Work out the finished part from the listing and answer in its coordinate system (mm). A direction names the side the tool comes from. Round coordinates to 2 decimals unless told otherwise and drop trailing zeros. Loops run counter-clockwise (first coordinate to the right, second up) from the corner with the lowest first, then second, coordinate; pieces in that order, holes last. Notation, with made-up numbers: (61, 26.25) - (66, 26.25) arc R21 cw to (66, 42.25) - close; hole circle Ø5 at (44, 19). An arc over 180 degrees is marked (long way). Use CSV: the item, a comma, the result in double quotes. Start each with the question number.
from build123d import *

# Parameters (mm, degrees)
BOSS_EXTRUDE1_DEPTH     = 22
BOSS_EXTRUDE3_START     = -5
BOSS_EXTRUDE3_OUTLINE_R = 1.5
BOSS_EXTRUDE3_DEPTH     = 5
CHAMFER2_SIZE           = 1
CHAMFER3_SIZE           = 7
CHAMFER3_SIZE2          = 2


# Read off the part's stored shape, not the designer's step: Boss-Extrude3
with BuildPart() as part:
    # Sketch1 → Boss-Extrude1 (new body)
    with BuildSketch(Plane(origin=(0, 0, 0), x_dir=(1, 0, 0), z_dir=(0, 1, 0))):
        with BuildLine():
            Line((0, -16.5), (0, -8.075))
            ThreePointArc((3.5438e-13, -8.075), (-5.709887258081245, -5.709887258081495), (-8.075, 1.03e-15))
            Line((-8.075, 0), (-16.5, 0))
            Line((-16.5, 0), (-24.5, -9.8e-16))
            Line((-24.5, -9.8e-16), (-24.5, -5.000000000000001))
            Line((-24.5, -5.000000000000001), (-15.724185193516389, -5.000000000000001))
            ThreePointArc((-15.724185193516387, -5), (-9.740379869388931, -13.318220601867306), (3.5527e-13, -16.5))
        make_face()
        with BuildLine():
            Line((24.5, -9.8e-16), (16.5, 0))
            Line((16.5, 0), (8.075, 0))
            ThreePointArc((8.075, 3.34e-15), (5.709887258081497, -5.709887258081244), (3.5438e-13, -8.075))
            Line((0, -8.075), (0, -16.5))
            ThreePointArc((3.5527e-13, -16.5), (9.74037986938922, -13.3182206018671), (15.724185193516387, -5.000000000000004))
            Line((15.724185193516389, -5.000000000000001), (24.5, -5.000000000000001))
            Line((24.5, -5.000000000000001), (24.5, -9.8e-16))
        make_face()
    extrude(amount=-BOSS_EXTRUDE1_DEPTH)

    # Boss-Extrude3 outline → Boss-Extrude3 (cut)
    with BuildSketch(Plane.XY.offset(5.000000000000001).offset(BOSS_EXTRUDE3_START)):
        with Locations((20.5, -18)):
            Circle(BOSS_EXTRUDE3_OUTLINE_R)
        with Locations((20.5, -4)):
            Circle(BOSS_EXTRUDE3_OUTLINE_R)
        with Locations((-20.5, -4)):
            Circle(BOSS_EXTRUDE3_OUTLINE_R)
        with Locations((-20.5, -18)):
            Circle(BOSS_EXTRUDE3_OUTLINE_R)
    extrude(amount=BOSS_EXTRUDE3_DEPTH, mode=Mode.SUBTRACT)

    # Chamfer2
    chamfer2_edges = [part.edges().sort_by_distance(p)[0] for p in [
        (-22, -18, 5.000000000000001),
        (19, -4, 5.000000000000001),
        (19, -18, 5.000000000000001),
        (-22, -4, 5.000000000000001),
    ]]
    chamfer(chamfer2_edges, length=CHAMFER2_SIZE)

    # Chamfer3
    chamfer3_edges = [part.edges().sort_by_distance(p)[0] for p in [
        (1.54e-15, -22, 8.075),
    ]]
    chamfer3_side = [part.faces().sort_by_distance(p)[0] for p in [
        (2.05e-15, -11, 8.075),
    ]]
    chamfer(chamfer3_edges, length=CHAMFER3_SIZE, length2=CHAMFER3_SIZE2, reference=chamfer3_side[0])

    # Sketch4 → Cut-Revolve1 (revolve, cut)
    with BuildSketch(Plane(origin=(0, 0, 0), x_dir=(-1, 0, -1.2e-16), z_dir=(1.2e-16, 0, -1))):
        with BuildLine():
            Line((-9.575, 0.4703111185771576), (-9.575, -1.4999999999999998))
            ThreePointArc((-9.575, -1.4999999999999998), (-7.014339828220178, -2.560660171779821), (-8.075, 0))
            Line((-8.075, 0), (-9.575, 0.4703111185771576))
        make_face()
    revolve(axis=Axis((4.3e-16, 1.8602118411515838, 0), (-1.7e-16, -1, 0)), mode=Mode.SUBTRACT)


solid = part.part
Item 1: The mould has two halves that part along X. Classify faces 3 (the flat face through (0, 0, 10)), 4 (the conical face through (0.195, -17.771, 8.865)), 5 (the flat face through (24.5, -11, 3)): pulls with the +X half, pulls with the -X half, needs draft (parallel to the pull), parting line crosses it, or undercut.
Item 2: A cutting plane is placed at B-B (x = 20.5). Determine the outline of the cut face in (y, z), plus the area to 3 significant figures.
Item 3: Find the intervals of material crossed by probe 1 along Y at (x, z) = (-20.5, 3.1); probe 2 along Z at (x, y) = (19, -7); probe 3 along X at (y, z) = (-1, 6), in increasing order. Write a range as [from, to].
Item 4: A cutting plane is placed at D-D (x = -17.5). Determine the outline of the cut face in (y, z), plus the area to 3 significant figures.
Item 5: Which of the six approach directions +Z, -Z, +X, -X, +Y, -Y give full straight-line access (tool end or side, diameter ignored) to faces 1 (the flat face through (20, -11, 5)), 2 (the flat face through (0, -22, 12))?
Item 6: A cutting plane is placed at C-C (y = -9.25). Determine the outline of the cut face in (x, z) (3 decimals).
Item 7: Each of these flat-tipped pins is pushed along its axis until it touches: pin 1 Ø3.5 at (x, y) = (20.5, -18) entering from +Z; pin 2 Ø6 at (x, y) = (-15.5, -7.5) entering from +Z; pin 3 Ø9.5 at (x, y) = (-19, -16) entering from +Z. Where does it stop, or does it pass through?
Item 8: A cutting plane is placed at A-A (y = -4). Determine the outline of the cut face in (x, z) (3 decimals).
Result sheet:
1,face 3,"needs draft"
1,face 4,"undercut"
1,face 5,"pulls with the +X half"
2,outline,"(-22, 0) - (-19.5, 0) - (-19.5, 4) - (-20.5, 5) - (-22, 5) - close; (-16.5, 0) - (-5.5, 0) - (-5.5, 4) - (-6.5, 5) - (-15.5, 5) - (-16.5, 4) - close; (-2.5, 0) - (0, 0) - (0, 5) - (-1.5, 5) - (-2.5, 4) - close"
2,area,"78.0 mm^2"
3,probe 1,"[-22, -19.5], [-16.5, -5.5], [-2.5, 0]"
3,probe 2,"[0, 5]"
3,probe 3,"[-15.37, -7.46], [7.46, 15.37]"
4,outline,"(-22, 0) - (0, 0) - (0, 5) - (-22, 5) - close"
4,area,"110 mm^2"
5,face 1,"+Z, +X, +Y, -Y"
5,face 2,"+Z, -Z, +X, -X, -Y"
6,outline,"(-24.5, 0) - (-8.075, 0) arc R8.075 cw to (8.075, 0) - (24.5, 0) - (24.5, 5) - (15.724, 5) arc R16.5 ccw to (-15.724, 5) - (-24.5, 5) - close"
7,pin 1,"z = 4.25"
7,pin 2,"z = 10.77"
7,pin 3,"z = 8.32"
8,outline,"(-24.5, 0) - (-22, 0) - (-22, 4) - (-23, 5) - (-24.5, 5) - close; (-19, 0) - (-8.075, 0) arc R8.075 cw to (8.075, 0) - (19, 0) - (19, 4) - (18, 5) - (15.724, 5) arc R16.5 ccw to (-15.724, 5) - (-18, 5) - (-19, 4) - close; (22, 0) - (24.5, 0) - (24.5, 5) - (23, 5) - (22, 4) - close"
